The listing builds one solid part. Answer for the finished solid, in the listing's coordinates (mm). A direction names the side the tool comes from. Coordinates: 2 decimals unless noted, no trailing zeros. Loops run counter-clockwise (first coordinate to the right, second up) from the corner with the lowest first, then second, coordinate; pieces in that order, holes last. Notation, with made-up numbers: (6, 10) - (27, 10) arc R17 cw to (27, 36) - close; hole circle Ø6 at (-16, -34). An arc over 180 degrees is marked (long way). Write each question's results on one line, items separated by ' | '. Start each with the question number.
(1) Find section A-A on z = -11.5. Determine the outline of the cut face in (x, y).
(2) Consider line 1 (X direction, y = 9, z = -6); line 2 (X direction, y = 9, z = 5.5); line 3 (X direction, y = 10.75, z = -8.5). Determine where each line is inside the solid, lowest interval first. Write a range as from..to.
(3) Given pin 1 Ø1 at (x, z) = (-38.5, 17.5) entering from -Y; pin 2 Ø1 at (x, z) = (-9, -9) entering from +Y; pin 3 Ø3.5 at (x, z) = (-6.5, -8) entering from +Y, each flat-ended and moving along its own axis, determine where each tip first touches the part or whether it passes through.
(4) Find section B-B on x = -41.5. Determine the outline of the cut face in (y, z), then the cut area to 3 significant figures.
(5) Find section C-C on z = -0.5. Determine the outline of the cut face in (x, y), then the cut area to 3 significant figures.
(6) For faces 1 (the flat face through (-1, 0, 0)), 2 (the flat face through (-7, 10, 11.5)), 3 (the cylindrical face through (-45, 10, 10.4)), determine the directions among +Z, -Z, +X, -X, +Y, -Y from which every point of the face is accessible in a straight line to the end or side of a thin tool.
(7) Determine the mould class of faces 4 (the cylindrical face through (0.7, 19.43, 21.9)), 5 (the cylindrical face through (0.7, 0.37, -17.32)), 6 (the flat face through (-7, 13, 17)) for opening direction Z: released by +Z, released by -Z, zero draft, split by the parting line, or undercut.
from build123d import *

# Parameters (mm, degrees)
SKETCH1_W           = 100
SKETCH1_H           = 45
BOSS_EXTRUDE1_DEPTH = 20
SHELL1_T            = -3
CHAMFER1_SIZE       = 5
FILLET1_R           = 5
SKETCH2_R           = 5.75
SKETCH2_R_2         = 3.25
CUT_EXTRUDE1_DEPTH  = 20
SKETCH3_R           = 1.5
CUT_EXTRUDE2_DEPTH  = 10
BOSS_EXTRUDE2_DEPTH = 3
FILLET2_R           = 1
SKETCH5_W           = 3
SKETCH5_H           = 39
BOSS_EXTRUDE3_DEPTH = 10
SKETCH6_W           = 3
SKETCH6_H           = 3
CUT_EXTRUDE3_DEPTH  = 5
FILLET3_R           = 1
FILLET4_R           = 2
FILLET6_R           = 0.5


with BuildPart() as part:
    # Sketch1 → Boss-Extrude1 (new body)
    with BuildSketch(Plane(origin=(0, 0, 0), x_dir=(1, 0, 0), z_dir=(0, 1, 0))):
        Rectangle(SKETCH1_W, SKETCH1_H)
    extrude(amount=BOSS_EXTRUDE1_DEPTH)

    # Shell1
    shell1_openings = [part.faces().sort_by_distance(p)[0] for p in [
        (0, 20, 0),
    ]]
    offset(amount=SHELL1_T, openings=shell1_openings, kind=Kind.INTERSECTION)

    # Chamfer1
    chamfer1_edges = [part.edges().sort_by_distance(p)[0] for p in [
        (0, 0, 22.5),
        (0, 0, -22.5),
    ]]
    chamfer(chamfer1_edges, length=CHAMFER1_SIZE)

    # Fillet1
    fillet1_edges = [part.edges().sort_by_distance(p)[0] for p in [
        (0, 5, -22.5),
        (0, 0, 17.5),
        (0, 0, -17.5),
        (0, 5, 22.5),
    ]]
    fillet(fillet1_edges, radius=FILLET1_R)

    # Sketch2 → Cut-Extrude1 (cut)
    with BuildSketch(Plane.ZY.offset(50)):
        with Locations((-11.5, 12)):
            Circle(SKETCH2_R)
        with Locations((10.5, 14)):
            Circle(SKETCH2_R_2)
    extrude(amount=-CUT_EXTRUDE1_DEPTH, mode=Mode.SUBTRACT)

    # Sketch3 → Cut-Extrude2 (cut)
    with BuildSketch(Plane.ZY.offset(50)):
        with Locations((13, 5)):
            Circle(SKETCH3_R)
    extrude(amount=-CUT_EXTRUDE2_DEPTH, mode=Mode.SUBTRACT)

    # Sketch4 → Boss-Extrude2 (add)
    with BuildSketch(Plane(origin=(-47, 0, 0), x_dir=(0, 0, -1), z_dir=(1, 0, 0))):
        with BuildLine():
            Line((5.733718703, 15), (6.594645782, 15))
            ThreePointArc((6.594645782, 15), (11.5, 6.25), (16.405354218, 15))
            Line((16.405354218, 15), (17.266281297, 15))
            ThreePointArc((17.266281297, 15), (11.5, 5.5), (5.733718703, 15))
        make_face()
        with BuildLine():
            Line((-14.372983346, 15), (-13.592329219, 15))
            ThreePointArc((-13.592329219, 15), (-10.5, 10.75), (-7.407670781, 15))
            Line((-7.407670781, 15), (-6.627016654, 15))
            ThreePointArc((-6.627016654, 15), (-10.5, 10), (-14.372983346, 15))
        make_face()
    extrude(amount=BOSS_EXTRUDE2_DEPTH)

    # Fillet2
    fillet2_edges = [part.edges().sort_by_distance(p)[0] for p in [
        (-47, 5.5, -11.5),
        (-47, 10, 10.5),
    ]]
    fillet(fillet2_edges, radius=FILLET2_R)

    # Sketch5 → Boss-Extrude3 (add)
    with BuildSketch(Plane(origin=(0, 3, 0), x_dir=(1, 0, 0), z_dir=(0, 1, 0))):
        with Locations((-6.5, 0)):
            Rectangle(SKETCH5_W, SKETCH5_H)
    extrude(amount=BOSS_EXTRUDE3_DEPTH)

    # Sketch6 → Cut-Extrude3 (cut)
    with BuildSketch(Plane(origin=(0, 13, 0), x_dir=(1, 0, 0), z_dir=(0, 1, 0))):
        with Locations((-6.5, -13)):
            Rectangle(SKETCH6_W, SKETCH6_H)
    extrude(amount=-CUT_EXTRUDE3_DEPTH, mode=Mode.SUBTRACT)

    # Fillet3
    fillet3_edges = [part.edges().sort_by_distance(p)[0] for p in [
        (-6.5, 13, 14.5),
        (-6.5, 13, 11.5),
    ]]
    fillet(fillet3_edges, radius=FILLET3_R)

    # Fillet4
    fillet4_edges = [part.edges().sort_by_distance(p)[0] for p in [
        (-50, 20, 0),
        (0, 20, 22.5),
        (50, 20, 0),
        (0, 20, -22.5),
    ]]
    fillet(fillet4_edges, radius=FILLET4_R)

    # Fillet6
    fillet6_edges = [part.edges().sort_by_distance(p)[0] for p in [
        (-50, 5, 11.5),
    ]]
    fillet(fillet6_edges, radius=FILLET6_R)


solid = part.part
Values:
1) outline: (-50, 0) - (50, 0) - (50, 18) arc R2 ccw to (48, 20) - (47, 20) - (47, 3) - (-5, 3) - (-5, 13) - (-8, 13) - (-8, 3) - (-47, 3) - (-47, 4.5) arc R1 cw to (-46, 5.5) - (-44, 5.5) - (-44, 6.25) - (-50, 6.25) - close; (-50, 17.75) - (-47, 17.75) - (-47, 20) - (-48, 20) arc R2 ccw to (-50, 18) - close
2) line 1: x = -50..-44, -8..-5, 47..50 | line 2: x = -50..-47, -8..-5, 47..50 | line 3: x = -8..-5, 47..50
3) pin 1: stops at y = 0.25 | pin 2: stops at y = 3 | pin 3: stops at y = 13
4) outline: (0, -15.43) arc R5 ccw to (1.46, -18.96) - (3.54, -21.04) arc R5 ccw to (7.07, -22.5) - (18, -22.5) arc R2 ccw to (20, -20.5) - (20, -19.5) - (3, -19.5) - (3, 19.5) - (20, 19.5) - (20, 20.5) arc R2 ccw to (18, 22.5) - (7.07, 22.5) arc R5 ccw to (3.54, 21.04) - (1.46, 18.96) arc R5 ccw to (0, 15.43) - close | area: 208 mm²
5) outline: (-50, 0) - (50, 0) - (50, 18) arc R2 ccw to (48, 20) - (47, 20) - (47, 3) - (-5, 3) - (-5, 13) - (-8, 13) - (-8, 3) - (-47, 3) - (-47, 20) - (-48, 20) arc R2 ccw to (-50, 18) - close | area: 430 mm²
6) face 1: +Z, -Z, +X, -X, -Y | face 2: +Y | face 3: none
7) face 4: released by +Z | face 5: released by -Z | face 6: undercut
